The listing builds one solid part. Answer for the finished solid, in the listing's coordinates (mm). Face numbers are marked on the shaded views. Coordinates: 2 decimals unless noted, no trailing zeros. Order: outer loops, then holes, each group sorted by start corner. A loop starts at its lowest first (then second) coordinate and runs counter-clockwise, first axis right, second up. Notation, with made-up numbers: (-20, 16.5) -> (21, 16.5) arc R18 ccw to (21, 29.5) -> close; hole circle Ø4 at (-0.75, 45). An arc over 180 degrees is marked (long way). Return JSON: item names as keys, results as strings.
Autodesk Inventor part; units mm, degrees
ref_plane "作業平面1" through (50.5, 0, 0) normal (1, 0, 0) x (0, 1, 0)
ref_plane "作業平面2" through (-50.5, 0, 0) normal (1, 0, 0) x (0, 1, 0)
ref_plane "作業平面3" through (0, 50.5, 0) normal (0, 1, 0) x (-1, 0, 0)
sketch "スケッチ1" plane through (0, 0, 0) normal (0, 0, 1) x (1, 0, 0)
  circle A0 centre (0, 0) radius 50.5
  dimension "d0" = 101
extrude "押し出し1" add sketch "スケッチ1" along normal blind 8
ref_plane "作業平面1" through (50.5, 0, 0) normal (1, 0, 0) x (0, 1, 0)
ref_plane "作業平面2" through (-50.5, 0, 0) normal (1, 0, 0) x (0, 1, 0)
ref_plane "作業平面3" through (0, 50.5, 0) normal (0, 1, 0) x (-1, 0, 0)
ref_plane "作業平面4" through (0, -50.5, 0) normal (0, 1, 0) x (-1, 0, 0)
sketch "スケッチ2" plane through (50.5, 0, 0) normal (1, 0, 0) x (0, 1, 0)
  line L0 (0, 0) -> (0, 4) construction
  circle A0 centre (0, 4) radius 1.5
  dimension "d7" = 4
  dimension "d8" = 3
extrude "押し出し2" cut sketch "スケッチ2" against normal blind 5
sketch "スケッチ3" plane through (-50.5, 0, 0) normal (1, 0, 0) x (0, 1, 0)
  line L0 (0, 0) -> (0, 4) construction
  circle A0 centre (0, 4) radius 1.5
  dimension "d11" = 4
  dimension "d12" = 3
extrude "押し出し3" cut sketch "スケッチ3" along normal blind 5
sketch "スケッチ4" plane through (0, 50.5, 0) normal (0, 1, 0) x (-1, 0, 0)
  line L0 (0, 0) -> (0, 4) construction
  circle A0 centre (0, 4) radius 1.5
  dimension "d15" = 4
  dimension "d16" = 3
extrude "押し出し4" cut sketch "スケッチ4" against normal blind 5
sketch "スケッチ5" plane through (0, -50.5, 0) normal (0, 1, 0) x (-1, 0, 0)
  line L0 (0, 0) -> (0, 4) construction
  circle A0 centre (0, 4) radius 1.5
  dimension "d19" = 4
  dimension "d20" = 3
extrude "押し出し5" cut sketch "スケッチ5" along normal blind 5
thread "ねじ1"
thread "ねじ2"
thread "ねじ3"
thread "ねじ4"
sketch "スケッチ8" plane through (0, 0, 8) normal (0, 0, 1) x (1, 0, 0)
  line L0 (0, 0) -> (0, 18.5) construction
  line L1 (0, 0) -> (0, -18.5) construction
  circle A0 centre (0, 18.5) radius 2
  circle A1 centre (0, -18.5) radius 2
  circle A2 centre (0, 0) radius 6.5
  dimension "d62" = 18.5
  dimension "d63" = 18.5
  dimension "d64" = 4
  dimension "d65" = 4
  dimension "d66" = 13
extrude "押し出し7" cut sketch "スケッチ8" against normal blind 8
thread "ねじ7"
thread "ねじ8"
sketch "スケッチ9" plane through (0, 0, 8) normal (0, 0, 1) x (1, 0, 0)
  line L0 (0, 0) -> (25, 0) construction
  line L1 (25, 0) -> (25, -1) construction
  line L2 (25, 0) -> (25, 7.5) construction
  circle A0 centre (36, 7.5) radius 1
  line L3 (36, 7.5) -> (14, 7.5) construction
  circle A1 centre (14, 7.5) radius 1
  line L4 (25, -1) -> (25, -10) construction
  line L5 (25, -10) -> (25, -28) construction
  circle A2 centre (11.5, -28) radius 1
  line L6 (25, 0) -> (9, 0) construction
  line L7 (9, 0) -> (9, -31) construction
  line L8 (9, -31) -> (41, -31) construction
  line L9 (41, -31) -> (41, 0) construction
  line L10 (25, 0) -> (25, 12) construction
  line L11 (14.417, 12) -> (35.583, 12) construction
  arc A3 (14.757, 12.2915) -> (9, 0) centre (25, 0) ccw construction
  arc A4 (41, 0) -> (35.583, 12) centre (25, 0) ccw construction
  line L12 (11.5, -28) -> (38.5, -28) construction
  circle A5 centre (38.5, -28) radius 1
  dimension "d92" = 25
  dimension "d103" = 7.5
  dimension "d105" = 2
  dimension "d108" = 2
  dimension "d117" = 2
  dimension "d129" = 16
  dimension "d130" = 31
  dimension "d131" = 32
  dimension "d134" = 22
  dimension "d146" = 28
  dimension "d147" = 27
  dimension "d148" = 2
extrude "押し出し11" cut sketch "スケッチ9" against normal blind 8
properties part number "outsideCover"
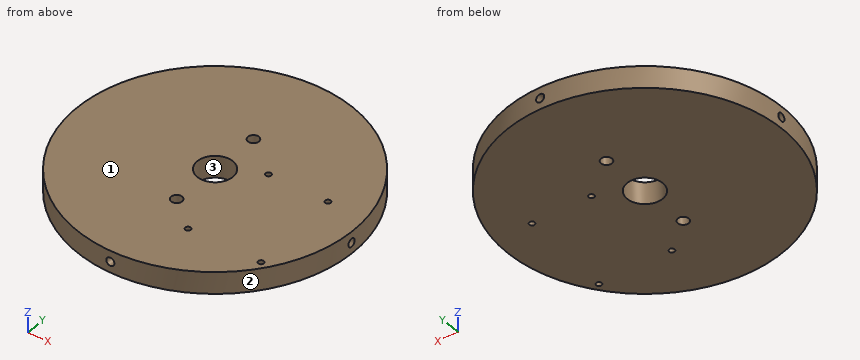
1. The part is cut by section C-C on x = 18.5. Give the vertices of the cut face in (y, z).
Answer block:
{"outline": "(-46.99, 0) -> (46.99, 0) -> (46.99, 8) -> (-46.99, 8) -> close"}
2. Determine the mould class of the marked faces 1, 2 and 3 for opening direction Y: pulls with the +Y half, pulls with the -Y half, needs draft (parallel to the pull), parting line crosses it, or undercut.
Answer block:
{"face 1": "needs draft", "face 2": "parting line crosses it", "face 3": "undercut"}
3. Each of these flat-tipped pins is pushed along its axis until it touches: pin 1 Ø1.5 at (x, z) = (0.5, 3.5) entering from +Y; pin 2 Ø3.5 at (x, y) = (0, -18.5) entering from -Z; pin 3 Ø1 at (x, z) = (-12.5, 4) entering from -Y; pin 4 Ø4 at (x, z) = (-35.5, 1) entering from -Y. Where does it stop, or does it pass through?
Answer block:
{"pin 1": "stops at y = 45.5", "pin 2": "passes through", "pin 3": "stops at y = -49.05", "pin 4": "stops at y = -37.79"}
4. The part is cut by section B-B on z = 4. Give the vertices of the cut face in (x, y).
Answer block:
{"outline": "(-50.48, -1.5) arc R50.5 ccw to (-1.5, -50.48) -> (-1.5, -45.5) -> (1.5, -45.5) -> (1.5, -50.48) arc R50.5 ccw to (50.48, -1.5) -> (45.5, -1.5) -> (45.5, 1.5) -> (50.48, 1.5) arc R50.5 ccw to (1.5, 50.48) -> (1.5, 45.5) -> (-1.5, 45.5) -> (-1.5, 50.48) arc R50.5 ccw to (-50.48, 1.5) -> (-45.5, 1.5) -> (-45.5, -1.5) -> close; hole circle Ø13 at (0, 0); hole circle Ø4 at (0, -18.5); hole circle Ø4 at (0, 18.5); hole circle Ø2 at (11.5, -28); hole circle Ø2 at (14, 7.5); hole circle Ø2 at (36, 7.5); hole circle Ø2 at (38.5, -28)"}
5. Consider line 1 (Y direction, x = 0, z = 2.25); line 2 (Y direction, x = 3, z = 4); line 3 (Y direction, x = 46.5, z = 4). Determine where each line is inside the solid, lowest interval first. Write a range as from..to.
Answer block:
{"line 1": "y = -50.5..-20.5, -16.5..-6.5, 6.5..16.5, 20.5..50.5", "line 2": "y = -50.41..-5.77, 5.77..50.41", "line 3": "y = -19.7..-1.5, 1.5..19.7"}
6. The part is cut by section A-A on y = 0. Give the vertices of the cut face in (x, z), and give its area (3 significant figures).
Answer block:
{"outline": "(-50.5, 0) -> (-6.5, 0) -> (-6.5, 8) -> (-50.5, 8) -> (-50.5, 5.5) -> (-45.5, 5.5) -> (-45.5, 2.5) -> (-50.5, 2.5) -> close; (6.5, 0) -> (50.5, 0) -> (50.5, 2.5) -> (45.5, 2.5) -> (45.5, 5.5) -> (50.5, 5.5) -> (50.5, 8) -> (6.5, 8) -> close", "area": "674 mm2"}
7. The part is cut by section D-D on y = -44. Give the vertices of the cut face in (x, z).
Answer block:
{"outline": "(-24.78, 0) -> (24.78, 0) -> (24.78, 8) -> (-24.78, 8) -> close"}
